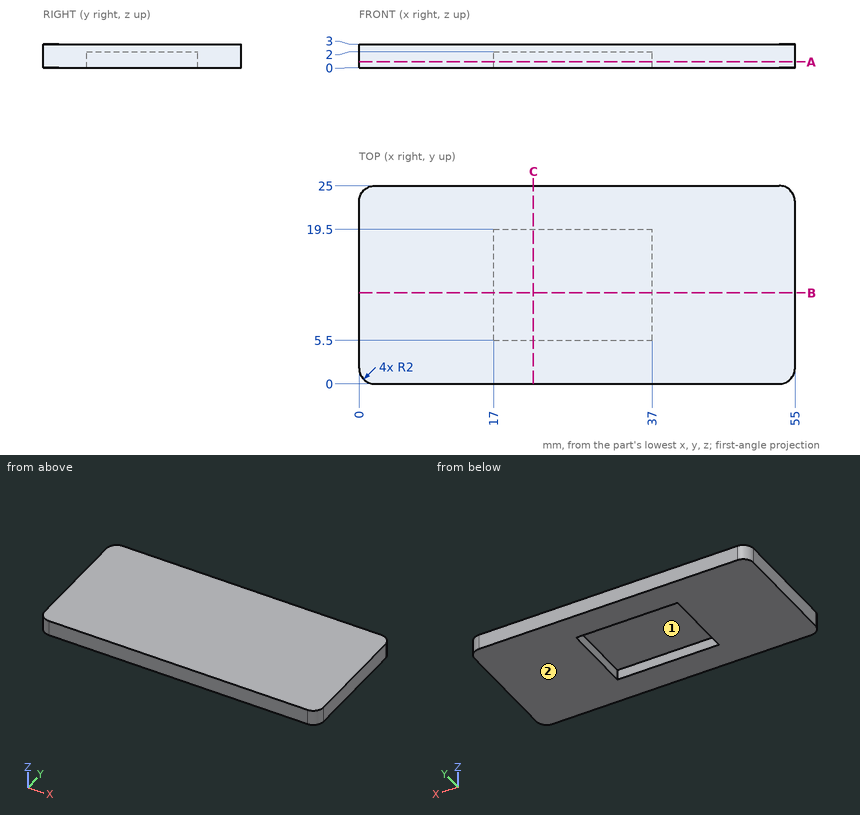
The figure shows three views and two pictorial views of one solid part (mm, origin at its lowest corner). Answer the questions. Give positions to 0.01 mm unless a question says otherwise; leave off trailing zeros. Order: outer loops, then holes, each group sorted by start corner. A loop starts at its lowest first (then second) coordinate and runs counter-clockwise, first axis right, second up. Notation, with made-up numbers: M 49,84.5 L 105,84.5 A31 cw 105,119.5 Z; hole C 43.5,54.25 d5. An arc over 180 degrees is marked long. Return JSON: item names as keys, results as strings.
Q1. Find section C-C, the plane x = 22. Write down the section's boundary in (y, z).
Answer below:
{"outline": "M 0,0 L 5.5,0 L 5.5,2 L 19.5,2 L 19.5,0 L 25,0 L 25,3 L 0,3 Z"}
Q2. Find section A-A, the plane z = 0.75. Write down the section's boundary in (x, y).
Answer below:
{"outline": "M 0,2 A2 ccw 2,0 L 53,0 A2 ccw 55,2 L 55,23 A2 ccw 53,25 L 2,25 A2 ccw 0,23 Z; hole M 17,5.5 L 37,5.5 L 37,19.5 L 17,19.5 Z"}
Q3. The mould has two halves that part along Y. Classify the marked faces 1 and 2: pulls with the +Y half, pulls with the -Y half, needs draft (parallel to the pull), parting line crosses it, or undercut.
Answer below:
{"face 1": "undercut", "face 2": "needs draft"}
Q4. Find the intervals of material crossed by line 1 along X through (y, z) = (12, 1.65); line 2 along Y through (x, z) = (21, 0.4); line 3 along Z through (x, y) = (25.5, 17.25), in increasing order. Write a range as [from, to].
Answer below:
{"line 1": "x = [0, 17], [37, 55]", "line 2": "y = [0, 5.5], [19.5, 25]", "line 3": "z = [2, 3]"}
Q5. Find section B-B, the plane y = 11.5. Write down the section's boundary in (x, z), and give its area (3 significant figures).
Answer below:
{"outline": "M 0,0 L 17,0 L 17,2 L 37,2 L 37,0 L 55,0 L 55,3 L 0,3 Z", "area": "125 mm^2"}
Q6. This flat-tipped pin is pushed along its axis until it touches: pin 1 (4 mm diameter, centred on x = 24.5, y = 13.5, fed in from -Z). Where does it stop, or does it pass through?
Answer below:
{"pin 1": "stops at z = 2"}
